Part print with two shaded views. Sizes in mm from the minimum x, y, z corner. A direction names the side the tool comes from. Round coordinates to 2 decimals unless told otherwise and drop trailing zeros. Loops run counter-clockwise (first coordinate to the right, second up) from the corner with the lowest first, then second, coordinate; pieces in that order, holes last.
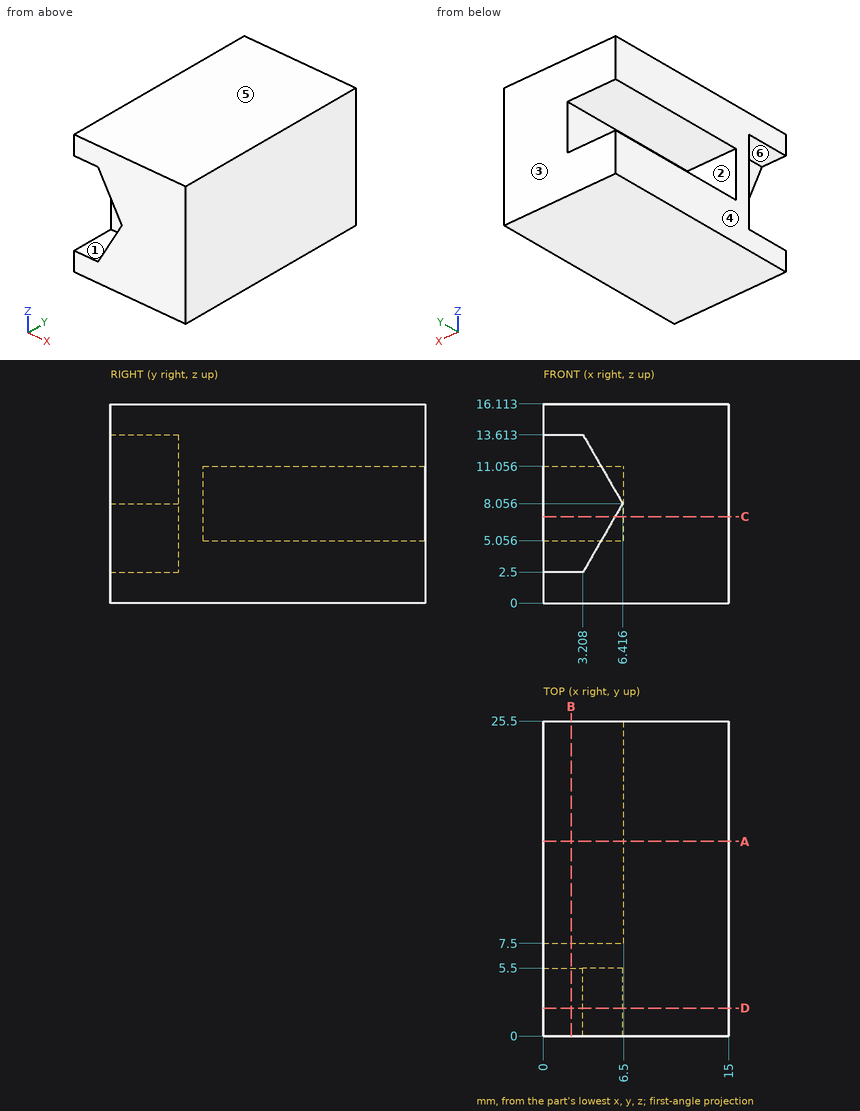
Item 1: Cut at B-B (x = 2.25). List the corners of the cut face in (y, z), plus the area to 3 significant figures.
Verdict:
outline: (0, 0) - (25.5, 0) - (25.5, 5.06) - (7.5, 5.06) - (7.5, 11.06) - (25.5, 11.06) - (25.5, 16.11) - (0, 16.11) - (0, 13.61) - (5.5, 13.61) - (5.5, 2.5) - (0, 2.5) - close
area: 242 mm2
Item 2: Mould opens along Z. For the marked faces 4, 5 and 6 say: released by +Z, released by -Z, zero draft, split by the parting line, or undercut.
Verdict:
face 4: zero draft
face 5: released by +Z
face 6: undercut
Item 3: Wall check: L1, parallel to Z at x = 3.5, y = 14; L2, parallel to X at y = 20.75, z = 11; L3, parallel to Y at x = 1.5, z = 8.5. Give the ranges that are in metal, low to high.
Verdict:
L1: z = 0 to 5.06, 11.06 to 16.11
L2: x = 6.5 to 15
L3: y = 5.5 to 7.5
Item 4: Flat gauge pins, fed straight in: P1, Ø7, axis at x = 1.5, z = 8.5, coming from the -Y side; P2, Ø5, axis at x = 2.5, z = 8.5, coming from the +Y side. Where does each tip first touch, or does it go through?
Verdict:
P1: stops at y = 5.5
P2: stops at y = 7.5
Item 5: Cut at C-C (z = 7). List the corners of the cut face in (x, y) (1 decimal).
Verdict:
outline: (0, 5.5) - (5.8, 5.5) - (5.8, 0) - (15, 0) - (15, 25.5) - (6.5, 25.5) - (6.5, 7.5) - (0, 7.5) - close
Item 6: 3-axis set-ups, long thin cutter, end or side, ignore diameter. For the marked faces 1, 2 and 3: which of +Z, -Z, +X, -X, +Y, -Y reach the whole face in a straight line?
Verdict:
face 1: -X, -Y
face 2: -X, +Y
face 3: +Z, -Z, +X, -X, +Y
Item 7: Cut at D-D (y = 2.25). List the corners of the cut face in (x, z) (1 decimal).
Verdict:
outline: (0, 0) - (15, 0) - (15, 16.1) - (0, 16.1) - (0, 13.6) - (3.2, 13.6) - (6.4, 8.1) - (3.2, 2.5) - (0, 2.5) - close
Item 8: Cut at A-A (y = 15.75). List the corners of the cut face in (x, z).
Verdict:
outline: (0, 0) - (15, 0) - (15, 16.11) - (0, 16.11) - (0, 11.06) - (6.5, 11.06) - (6.5, 5.06) - (0, 5.06) - close
